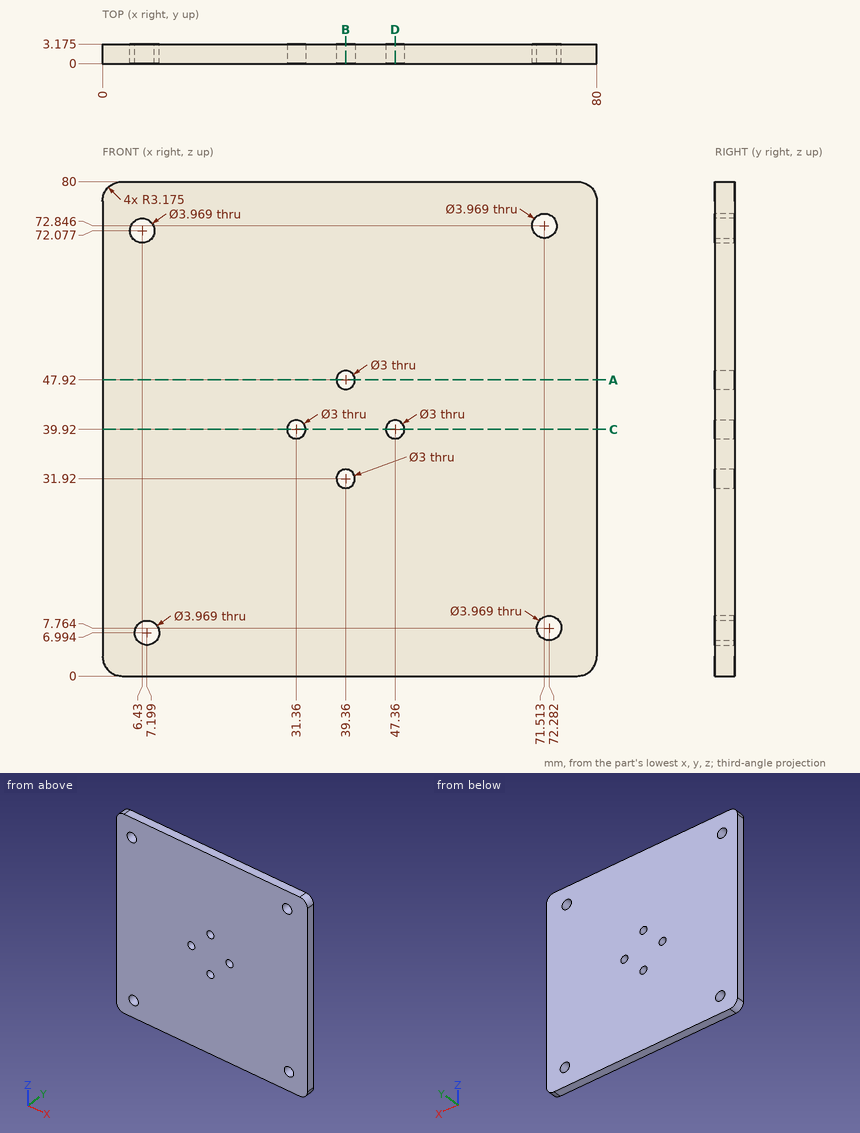
Geometry check sheet. Reference: drawing and pictorial views, mm from the part's lowest x, y, z. Round coordinates to 2 decimals unless told otherwise and drop trailing zeros. Order: outer loops, then holes, each group sorted by start corner. A loop starts at its lowest first (then second) coordinate and runs counter-clockwise, first axis right, second up.
Q1. Cross-section at A-A, the plane z = 47.92. Enter the section's corners in (x, y) (1 decimal).
Filled sheet:
outline: (0, 0) - (37.9, 0) - (37.9, 3.2) - (0, 3.2) - close; (40.9, 0) - (80, 0) - (80, 3.2) - (40.9, 3.2) - close
Q2. Cross-section at B-B, the plane x = 39.36. Enter the section's corners in (y, z) (1 decimal), plus the area to 3 significant figures.
Filled sheet:
outline: (0, 0) - (3.2, 0) - (3.2, 30.4) - (0, 30.4) - close; (0, 33.4) - (3.2, 33.4) - (3.2, 46.4) - (0, 46.4) - close; (0, 49.4) - (3.2, 49.4) - (3.2, 80) - (0, 80) - close
area: 235 mm2
Q3. Cross-section at C-C, the plane z = 39.92. Enter the section's corners in (x, y) (1 decimal).
Filled sheet:
outline: (0, 0) - (29.9, 0) - (29.9, 3.2) - (0, 3.2) - close; (32.9, 0) - (45.9, 0) - (45.9, 3.2) - (32.9, 3.2) - close; (48.9, 0) - (80, 0) - (80, 3.2) - (48.9, 3.2) - close
Q4. Cross-section at D-D, the plane x = 47.36. Enter the section's corners in (y, z) (1 decimal).
Filled sheet:
outline: (0, 0) - (3.2, 0) - (3.2, 38.4) - (0, 38.4) - close; (0, 41.4) - (3.2, 41.4) - (3.2, 80) - (0, 80) - close
Q5. Scan lines: L1, parallel to X at y = 1.95, z = 39.92; L2, parallel to Z at x = 72, y = 2.4; L3, parallel to Z at x = 72.5, y = 1.7 (1 decimal). Record each from-to range of solid material in increasing order.
Filled sheet:
L1: x = 0 to 29.86, 32.86 to 45.86, 48.86 to 80
L2: z = 0 to 5.8, 9.73 to 70.92, 74.77 to 80
L3: z = 0 to 5.8, 9.7 to 71.1, 74.6 to 80
